The model under review builds one solid part; all positions refer to its coordinate system, in mm. A direction names the side the tool comes from. Round coordinates to 2 decimals unless told otherwise and drop trailing zeros. Use a Markdown table: item, result. Add a question column.
1) Insertion check: pin 1 (2.5 mm diameter, centred on y = -29.5, z = 18, fed in from -X). The pin has a flat end and moves straight along its axis. Give the tip position at first contact, or say it passes through.
2) Mouldability with a two-part tool opening along Z and no side actions: class faces 4 (the cylindrical face through (24.711, -2.056, 17.059)), 5 (the flat face through (25, -32, 20.298)), 6 (the cylindrical face through (25.004, -67.435, 19.504)), 7 (the flat face through (26.799, -0.5, 17.9)) as released by +Z, released by -Z, zero draft, split by the parting line, or undercut.
3) For faces 1 (the flat face through (25, -65.088, 16)), 2 (the flat face through (25, -65.088, 20)), 3 (the flat face through (25, 0, 18)), list the 3-axis set-ups (+Z, -Z, +X, -X, +Y, -Y) from which the entire face can be reached by the end or side of a thin tool; tool diameter is ignored.
4) Wall thickness on probe 1 along Y at (x, z) = (25.35, 17.8); probe 2 along Y at (x, z) = (26.25, 20.1); probe 3 along X at (y, z) = (-63, 17.1): over which ranges is each line inside the solid? List them lowest first.
from build123d import *

# Parameters (mm, degrees)
F0_W           = 3.175
F0_H           = 4.7625
F1_DEPTH       = 65.0875
F2_R           = 1.6002
F3_DEPTH       = 4.7625
F5_D           = 2.8194
F5_CSINK_D     = 4.7625
F5_CSINK_ANGLE = 90


with BuildPart() as f1:
    # F0 (on Front) → F1 (new body)
    with BuildSketch(Plane.XZ):
        with Locations((25.211968, 17.917172)):
            Rectangle(F0_W, F0_H)
    extrude(amount=F1_DEPTH)

    # F2 (on face) → F3 (join)
    with BuildSketch(Plane.XZ.offset(65.0875)):
        with Locations((25.211968, 17.917172)):
            Circle(F2_R)
    extrude(amount=F3_DEPTH)

    # F5 (through all)
    with Locations(Plane.YZ.offset(26.799468)):
        with Locations((-3.175, 17.917172)):
            CounterSinkHole(F5_D / 2, F5_CSINK_D / 2, counter_sink_angle=F5_CSINK_ANGLE)


solid = f1.part
Result set:
| question | item | result |
|---|---|---|
| 1 | pin 1 | x = 23.62 |
| 2 | face 4 | undercut |
| 2 | face 5 | released by +Z |
| 2 | face 6 | split by the parting line |
| 2 | face 7 | zero draft |
| 3 | face 1 | -Z, -Y |
| 3 | face 2 | +Z, -Y |
| 3 | face 3 | +Z, -Z, +X, -X, +Y |
| 4 | probe 1 | -69.85 to -4.58, -1.77 to 0 |
| 4 | probe 2 | -65.09 to 0 |
| 4 | probe 3 | 23.62 to 26.8 |
